Can you work these out from the model? Positions are in its coordinate system, mm. A direction names the side the tool comes from. Round coordinates to 2 decimals unless told otherwise and drop trailing zeros. Write each loop counter-clockwise with the first axis right and the second up, starting at its lowest first coordinate (ties: lowest second). Pieces come first, ordered by that corner, then holes. Notation, with made-up numbers: M 18.5,-13 L 46.5,-13 A29 cw 46.5,8 Z; hole C 53.5,-40 d7. An arc over 180 degrees is marked long. Use one line per item in the form item = value. Start each with the question number.
```python
from build123d import *

# Parameters (mm, degrees)
PAD_DEPTH    = 10
SKETCH001_R  = 2
POCKET_DEPTH = 5


with BuildPart() as part:
    # Sketch → Pad (new body)
    with BuildSketch(Plane.XY):
        Polygon((34.6, 94.4), (-34.6, 94.4), (-34.6, 2.4), (-44.6, 2.4), (-44.6, 0), (-32.2, 0), (-32.2, 92), (32.2, 92), (32.2, 0), (44.6, 0), (44.6, 2.4), (34.6, 2.4), align=None)
    extrude(amount=PAD_DEPTH)

    # Sketch001 → Pocket (cut)
    with BuildSketch(Plane.XZ):
        with Locations((-37.5, 5)):
            Circle(SKETCH001_R)
        with Locations((37.5, 5)):
            Circle(SKETCH001_R)
    extrude(amount=-POCKET_DEPTH, mode=Mode.SUBTRACT)


solid = part.part
```
1. If we mould it in two halves opening along X, with no side actions, what happens to faces 4 (the face through (44.6, 1, 5)), 5 (the face through (-44.6, 1, 5)), 6 (the face through (-32.2, 45, 5))? For each: pulls with the +X half, pulls with the -X half, needs draft (parallel to the pull), parting line crosses it, or undercut.
2. If we section it at B-B (z = 5): List the corners of the cut face in (x, y) for me, and give its area (3 significant figures).
3. If we section it at D-D (x = -23.5): List the corners of the cut face in (y, z) for me.
4. Which directions (+Z, -Z, +X, -X, +Y, -Y) give clear straight access to the entire face, cutting with the end or side of a thin tool? Please do faces 1 (the face through (0, 92, 5)), 2 (the face through (34.6, 48, 5)), 3 (the face through (-40, 2.4, 5)).
5. If we section it at C-C (x = 37.5): List the corners of the cut face in (y, z) for me.
6. If we section it at A-A (y = 79): List the corners of the cut face in (x, z) for me.
7. Will these pins go through, and if not, where does the flat tip stop? pin 1 (1.5 mm diameter, centred on x = -35.5, z = 4, fed in from -Y); pin 2 (3.5 mm diameter, centred on x = 37.5, z = 5, fed in from -Y); pin 3 (3 mm diameter, centred on x = -40.5, z = 3.5, fed in from +Y); pin 4 (5 mm diameter, centred on y = 66, z = 2.5, fed in from -X).
8. Please list where these lines run through material, in increasing order: line 1 along X through (y, z) = (40.5, 9.25); line 2 along Z through (x, y) = (37.5, 1.4); line 3 along Y through (x, z) = (39, 2.5).
Model answer:
q1.face_4 = pulls with the +X half
q1.face_5 = pulls with the -X half
q1.face_6 = undercut
q2.outline = M -44.6,0 L -39.5,0 L -39.5,2.4 L -44.6,2.4 Z; M -35.5,0 L -32.2,0 L -32.2,92 L 32.2,92 L 32.2,0 L 35.5,0 L 35.5,2.4 L 34.6,2.4 L 34.6,94.4 L -34.6,94.4 L -34.6,2.4 L -35.5,2.4 Z; M 39.5,0 L 44.6,0 L 44.6,2.4 L 39.5,2.4 Z
q2.area = 636 mm2
q3.outline = M 92,0 L 94.4,0 L 94.4,10 L 92,10 Z
q4.face_1 = +Z, -Z, -Y
q4.face_2 = +Z, -Z, +X, +Y
q4.face_3 = +Z, -Z, -X, +Y
q5.outline = M 0,0 L 2.4,0 L 2.4,3 L 0,3 Z; M 0,7 L 2.4,7 L 2.4,10 L 0,10 Z
q6.outline = M -34.6,0 L -32.2,0 L -32.2,10 L -34.6,10 Z; M 32.2,0 L 34.6,0 L 34.6,10 L 32.2,10 Z
q7.pin_1 = 0
q7.pin_2 = through
q7.pin_3 = 2.4
q7.pin_4 = -34.6
q8.line_1 = -34.6 to -32.2, 32.2 to 34.6
q8.line_2 = 0 to 3, 7 to 10
q8.line_3 = 0 to 2.4
